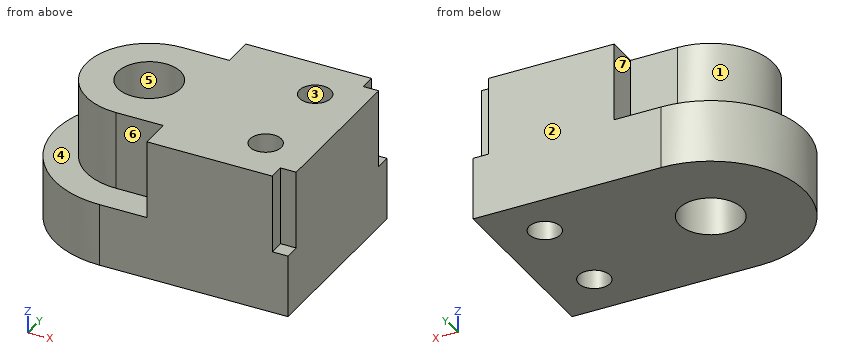
from build123d import *

# Parameters (mm, degrees)
PAD_DEPTH       = 45
SKETCH001_W     = 5
SKETCH001_H     = 5
POCKET_DEPTH    = 25
SKETCH002_R     = 10
SKETCH002_R_2   = 5
POCKET001_DEPTH = 45.001


with BuildPart() as part:
    # Sketch → Pad (new body)
    with BuildSketch(Plane.XY):
        with BuildLine():
            ThreePointArc((0, 30), (-30, 0), (0, -30))
            Line((60, -30), (0, -30))
            Line((60, 30), (60, -30))
            Line((0, 30), (60, 30))
        make_face()
    extrude(amount=PAD_DEPTH)

    # Sketch001 (on Face6 of Pad) → Pocket (cut)
    with BuildSketch(Plane.XY.offset(45)):
        with BuildLine():
            ThreePointArc((0, 20), (-20, 0), (0, -20))
            Line((0, -20), (15, -20))
            Line((15, -20), (15, -30))
            Line((15, -30), (0, -30))
            ThreePointArc((0, 30), (-30, 0), (0, -30))
            Line((0, 30), (15, 30))
            Line((15, 30), (15, 20))
            Line((15, 20), (0, 20))
        make_face()
        with Locations((57.5, 27.5)):
            Rectangle(SKETCH001_W, SKETCH001_H)
        with Locations((57.5, -27.5)):
            Rectangle(SKETCH001_W, SKETCH001_H)
    extrude(amount=-POCKET_DEPTH, mode=Mode.SUBTRACT)

    # Sketch002 (on Face8 of Pocket) → Pocket001 (cut, through all)
    with BuildSketch(Plane.XY.offset(45)):
        Circle(SKETCH002_R)
        with Locations((45, 15)):
            Circle(SKETCH002_R_2)
        with Locations((45, -15)):
            Circle(SKETCH002_R_2)
    extrude(amount=-POCKET001_DEPTH, mode=Mode.SUBTRACT)


solid = part.part
The listing builds one solid part. Answer for the finished solid, in the listing's coordinates (mm). Face numbers are marked on the shaded views. A direction names the side the tool comes from. Give positions to 0.01 mm unless a question says otherwise; leave off trailing zeros. Loops run counter-clockwise (first coordinate to the right, second up) from the corner with the lowest first, then second, coordinate; pieces in that order, holes last. Notation, with made-up numbers: (76, 38) - (133, 38) arc R27 ccw to (133, 69) - close; hole circle Ø5 at (3, 63.5). An arc over 180 degrees is marked (long way). Write each question's results on one line, items separated by ' | '.
1. Find section A-A, the plane y = 0. Write down the section's boundary in (x, z).
Resolved:
outline: (-30, 0) - (-10, 0) - (-10, 45) - (-20, 45) - (-20, 20) - (-30, 20) - close; (10, 0) - (60, 0) - (60, 45) - (10, 45) - close
2. Flat-ended cylindrical pins translate along their axes: P1, Ø2.5, axis at y = 28.5, z = 31, coming from the +X side; P2, Ø16.5, axis at x = 11, z = 37, coming from the -Y side; P3, Ø3, axis at x = -17.5, z = 36, coming from the +Y side; P4, Ø2.5, axis at x = 58, y = 26.5, coming from the +Z side. Find the tip coordinate at first contact, or state that the pin passes through.
Resolved:
P1: stops at x = 55 | P2: stops at y = -30 | P3: stops at y = 12 | P4: stops at z = 20
3. For a pull along Y with two mould halves and no side action, classify the marked faces 1, 2, 3 and 4 as +Y half, -Y half, draft (parallel to the pull), parting line (faces both ways), or undercut.
Resolved:
face 1: parting line | face 2: +Y half | face 3: undercut | face 4: draft
4. Which of the six approach directions +Z, -Z, +X, -X, +Y, -Y give full straight-line access (tool end or side, diameter ignored) to the marked faces 5, 6 and 7?
Resolved:
face 5: +Z, -Z | face 6: +Z, -X, -Y | face 7: +Z, -X, +Y
5. Find section C-C, the plane x = 45. Write down the section's boundary in (y, z), then the cut area to 3 significant figures.
Resolved:
outline: (-30, 0) - (-20, 0) - (-20, 45) - (-30, 45) - close; (-10, 0) - (10, 0) - (10, 45) - (-10, 45) - close; (20, 0) - (30, 0) - (30, 45) - (20, 45) - close | area: 1,800 mm^2
6. Find section D-D, the plane z = 21. Write down the section's boundary in (x, y), then the cut area to 3 significant figures.
Resolved:
outline: (0, -20) - (15, -20) - (15, -30) - (55, -30) - (55, -25) - (60, -25) - (60, 25) - (55, 25) - (55, 30) - (15, 30) - (15, 20) - (0, 20) arc R20 ccw to start; hole circle Ø20 at (0, 0); hole circle Ø10 at (45, -15); hole circle Ø10 at (45, 15) | area: 3,410 mm^2
7. Find section B-B, the plane z = 10.5. Write down the section's boundary in (x, y), then the cut area to 3 significant figures.
Resolved:
outline: (0, -30) - (60, -30) - (60, 30) - (0, 30) arc R30 ccw to start; hole circle Ø20 at (0, 0); hole circle Ø10 at (45, -15); hole circle Ø10 at (45, 15) | area: 4,540 mm^2
8. Consider probe 1 along Y at (x, z) = (45, 27); probe 2 along X at (y, z) = (-0.5, 26.5); probe 3 along Z at (x, y) = (-22, 6.5). Determine where each line is inside the solid, lowest interval first. Write a range as from..to.
Resolved:
probe 1: y = -30..-20, -10..10, 20..30 | probe 2: x = -19.99..-9.99, 9.99..60 | probe 3: z = 0..20
